For this review, take the finished solid that the model builds, in its own axes (mm). Give positions to 0.01 mm unless a question says otherwise; leave off trailing zeros. Order: outer loops, then holes, each group sorted by start corner. A loop starts at its lowest first (then second) coordinate and runs counter-clockwise, first axis right, second up.
from build123d import *

# Parameters (mm, degrees)
F0_R     = 1.55
F0_W     = 1.6
F0_H     = 5.1
F0_W_2   = 14
F0_H_2   = 14
F0_R_2   = 1.05
F0_R_3   = 3
F1_DEPTH = 1.5
F2_R     = 3
F3_R     = 1.5
F4_DEPTH = 1.501


with BuildPart() as f1:
    # F0 (on Top) → F1 (new body)
    with BuildSketch(Plane.XY):
        Polygon((18.45, -32), (16.45, -32), (-16.45, -32), (-18.45, -32), (-18.45, -58), (18.45, -58), align=None)
        Polygon((-16.45, -32), (16.45, -32), (16.45, -5.4752086141), (16.45, 13), (16.45, 32), (-16.45, 32), (-16.45, 13), (-16.45, -5.4752086141), align=None)
        with Locations((-14.2, -25)):
            Circle(F0_R, mode=Mode.SUBTRACT)
        with Locations((-10, -18)):
            Circle(F0_R, mode=Mode.SUBTRACT)
        with Locations((14.2, -25)):
            Circle(F0_R, mode=Mode.SUBTRACT)
        with Locations((10, -18)):
            Circle(F0_R, mode=Mode.SUBTRACT)
        with Locations((-10, 2)):
            Circle(F0_R, mode=Mode.SUBTRACT)
        with Locations((-14.2, 9)):
            Circle(F0_R, mode=Mode.SUBTRACT)
        with Locations((-14.2, 15.55)):
            Rectangle(F0_W, F0_H, mode=Mode.SUBTRACT)
        with Locations((-14.2, 26.45)):
            Rectangle(F0_W, F0_H, mode=Mode.SUBTRACT)
        with Locations((0, -8)):
            Rectangle(F0_W_2, F0_H_2, mode=Mode.SUBTRACT)
        with Locations((10, 2)):
            Circle(F0_R, mode=Mode.SUBTRACT)
        with Locations((14.2, 9)):
            Circle(F0_R, mode=Mode.SUBTRACT)
        Polygon((-10, 14), (0, 18), (10, 14), (10, 12), (0, 16), (-10, 12), align=None, mode=Mode.SUBTRACT)
        with Locations((14.2, 15.55)):
            Rectangle(F0_W, F0_H, mode=Mode.SUBTRACT)
        Polygon((-10, 19), (0, 23), (10, 19), (10, 17), (0, 21), (-10, 17), align=None, mode=Mode.SUBTRACT)
        Polygon((-10, 24), (0, 28), (10, 24), (10, 22), (0, 26), (-10, 22), align=None, mode=Mode.SUBTRACT)
        with Locations((14.2, 26.45)):
            Rectangle(F0_W, F0_H, mode=Mode.SUBTRACT)
        Polygon((16.45, -5.4752086141), (16.45, -32), (18.45, -32), (18.45, -4.3205080757), align=None)
        Polygon((-18.45, -32), (-16.45, -32), (-16.45, -5.4752086141), (-18.45, -4.3205080757), align=None)
        with BuildLine():
            Line((16.45, 13), (16.45, -5.4752086141))
            Line((16.45, -5.4752086141), (18.45, -4.3205080757))
            Line((18.45, -4.3205080757), (60.8230669589, 20.1435935394))
            ThreePointArc((60.8230669589, 20.1435935394), (63.7512701892, 31.0717967697), (52.8230669589, 34))
            Line((52.8230669589, 34), (16.45, 13))
        make_face()
        with Locations((55.2701526883, 21.276241812)):
            Circle(F0_R_2, mode=Mode.SUBTRACT)
        with Locations((51.0275120012, 28.6247110403)):
            Circle(F0_R_2, mode=Mode.SUBTRACT)
        with Locations((62.6186219167, 25.5188824991)):
            Circle(F0_R_2, mode=Mode.SUBTRACT)
        with Locations((56.8230669589, 27.0717967697)):
            Circle(F0_R_3, mode=Mode.SUBTRACT)
        with Locations((58.3759812296, 32.8673517275)):
            Circle(F0_R_2, mode=Mode.SUBTRACT)
        with BuildLine():
            Line((-18.45, -4.3205080757), (-16.45, -5.4752086141))
            Line((-16.45, -5.4752086141), (-16.45, 13))
            Line((-16.45, 13), (-52.8230669589, 34))
            ThreePointArc((-52.8230669589, 34), (-63.7512701892, 31.0717967697), (-60.8230669589, 20.1435935394))
            Line((-60.8230669589, 20.1435935394), (-18.45, -4.3205080757))
        make_face()
        with Locations((-55.2701526883, 21.276241812)):
            Circle(F0_R_2, mode=Mode.SUBTRACT)
        with Locations((-62.6186219167, 25.5188824991)):
            Circle(F0_R_2, mode=Mode.SUBTRACT)
        with Locations((-56.8230669589, 27.0717967697)):
            Circle(F0_R_3, mode=Mode.SUBTRACT)
        with Locations((-51.0275120012, 28.6247110403)):
            Circle(F0_R_2, mode=Mode.SUBTRACT)
        with Locations((-58.3759812296, 32.8673517275)):
            Circle(F0_R_2, mode=Mode.SUBTRACT)
    extrude(amount=F1_DEPTH)

    # F2
    f2_edges = [f1.edges().sort_by_distance(p)[0] for p in [
        (-16.45, 13, 0.75),
        (16.45, 13, 0.75),
        (18.45, -4.320508, 0.75),
        (-18.45, -4.320508, 0.75),
        (16.45, 32, 0.75),
        (-16.45, 32, 0.75),
    ]]
    fillet(f2_edges, radius=F2_R)

    # F3 (on face) → F4 (cut, through all)
    with BuildSketch(Plane.XY.offset(1.5)):
        with BuildLine():
            ThreePointArc((-12.95, -1), (-14.2, 0.25), (-15.45, -1))
            Line((-15.45, -1), (-15.45, -16))
            ThreePointArc((-15.45, -16), (-14.2, -17.25), (-12.95, -16))
            Line((-12.95, -16), (-12.95, -1))
        make_face()
        with BuildLine():
            ThreePointArc((15.45, -1), (14.2, 0.25), (12.95, -1))
            Line((12.95, -1), (12.95, -16))
            ThreePointArc((12.95, -16), (14.2, -17.25), (15.45, -16))
            Line((15.45, -16), (15.45, -1))
        make_face()
        with BuildLine():
            ThreePointArc((-12.95, -30), (-14.2, -28.75), (-15.45, -30))
            Line((-15.45, -30), (-15.45, -37))
            ThreePointArc((-15.45, -37), (-14.2, -38.25), (-12.95, -37))
            Line((-12.95, -37), (-12.95, -30))
        make_face()
        with BuildLine():
            ThreePointArc((15.45, -30), (14.2, -28.75), (12.95, -30))
            Line((12.95, -30), (12.95, -37))
            ThreePointArc((12.95, -37), (14.2, -38.25), (15.45, -37))
            Line((15.45, -37), (15.45, -30))
        make_face()
        with Locations((-14, -45)):
            Circle(F3_R)
        with Locations((-14, -53)):
            Circle(F3_R)
        with Locations((14, -45)):
            Circle(F3_R)
        with Locations((14, -53)):
            Circle(F3_R)
        with BuildLine():
            ThreePointArc((-6.2, -26.25), (-7.45, -27.5), (-6.2, -28.75))
            Line((-6.2, -28.75), (6.2, -28.75))
            ThreePointArc((6.2, -28.75), (7.45, -27.5), (6.2, -26.25))
            Line((6.2, -26.25), (-6.2, -26.25))
        make_face()
        with BuildLine():
            ThreePointArc((-6.2, -38.25), (-7.45, -39.5), (-6.2, -40.75))
            Line((-6.2, -40.75), (6.2, -40.75))
            ThreePointArc((6.2, -40.75), (7.45, -39.5), (6.2, -38.25))
            Line((6.2, -38.25), (-6.2, -38.25))
        make_face()
    extrude(amount=-F4_DEPTH, mode=Mode.SUBTRACT)


solid = f1.part
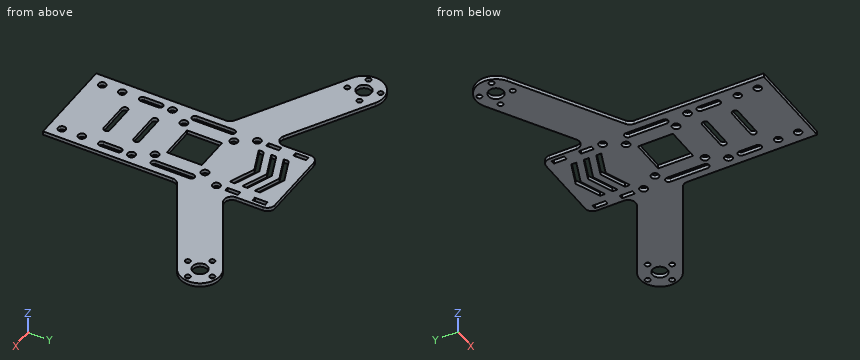
1) To check wall thickness, follow line 1 (X direction, y = -36, z = 0.25); line 2 (X direction, y = -41, z = 0.3). State the ranges of each line that lie inside material, in increasing order.
Answer sheet:
line 1: x = -18.45 to -15.45, -12.95 to 12.95, 15.45 to 18.45
line 2: x = -18.45 to 18.45
2) We need section A-A on y = -45. Give the boundary of the cut face in (x, z), then the cut area to 4 significant figures.
Answer sheet:
outline: (-18.45, 0) - (-15.5, 0) - (-15.5, 1.5) - (-18.45, 1.5) - close; (-12.5, 0) - (12.5, 0) - (12.5, 1.5) - (-12.5, 1.5) - close; (15.5, 0) - (18.45, 0) - (18.45, 1.5) - (15.5, 1.5) - close
area: 46.35 mm2
3) We need section B-B on x = -3. Give the boundary of the cut face in (y, z), then the cut area to 3 significant figures.
Answer sheet:
outline: (-58, 0) - (-40.75, 0) - (-40.75, 1.5) - (-58, 1.5) - close; (-38.25, 0) - (-28.75, 0) - (-28.75, 1.5) - (-38.25, 1.5) - close; (-26.25, 0) - (-15, 0) - (-15, 1.5) - (-26.25, 1.5) - close; (-1, 0) - (14.8, 0) - (14.8, 1.5) - (-1, 1.5) - close; (16.8, 0) - (19.8, 0) - (19.8, 1.5) - (16.8, 1.5) - close; (21.8, 0) - (24.8, 0) - (24.8, 1.5) - (21.8, 1.5) - close; (26.8, 0) - (32, 0) - (32, 1.5) - (26.8, 1.5) - close
area: 97.5 mm2
4) We need section D-D on y = 9. Give the boundary of the cut face in (x, z), then the cut area to 3 significant figures.
Answer sheet:
outline: (-41.52, 0) - (-15.75, 0) - (-15.75, 1.5) - (-41.52, 1.5) - close; (-12.65, 0) - (12.65, 0) - (12.65, 1.5) - (-12.65, 1.5) - close; (15.75, 0) - (41.52, 0) - (41.52, 1.5) - (15.75, 1.5) - close
area: 115 mm2
5) We need section C-C on z = 0.6. Count the separate pieces of the cut face and the enclosed holes in it, then the cut area to 3 significant figures.
Answer sheet:
separate pieces: 1
enclosed holes: 36
area: 4,150 mm2
6) Clearance check with flat-ended pins moving along their axes: pin 1 (0.8 mm diameter, centred on y = 12.5, z = 1, fed in from +X); pin 2 (0.8 mm diameter, centred on y = 26, z = 0.5, fed in from +X); pin 3 (0.8 mm diameter, centred on y = 25, z = 1, fed in from -X). State where each tip first meets the part, or that it passes through.
Answer sheet:
pin 1: stops at x = 48.28
pin 2: stops at x = 64.79
pin 3: stops at x = -64.65
